from build123d import *

# Parameters (mm, degrees)
SKETCH_1_R          = 1.75
EXTRUDE_1_DEPTH     = 1
SKETCH_2_W          = 5
SKETCH_2_H          = 3.5
SKETCH_2_W_2        = 2
SKETCH_2_H_2        = 6.5
CUT_EXTRUDE_1_DEPTH = 2
SKETCH_3_W          = 14.891608376
SKETCH_3_H          = 2
EXTRUDE_2_DEPTH     = 5
FILLET_1_R          = 2


with BuildPart() as part:
    # 草图1 → 凸台-拉伸1 (new body)
    with BuildSketch(Plane.XY):
        with BuildLine():
            Line((-7.445804188, 14.5), (7.445804188, 14.5))
            ThreePointArc((7.445804188, 14.5), (0, -16.3), (-7.445804188, 14.5))
        make_face()
        Circle(SKETCH_1_R, mode=Mode.SUBTRACT)
    extrude(amount=EXTRUDE_1_DEPTH)

    # 草图2 → 切除-拉伸1 (cut, through all)
    with BuildSketch(Plane.XY.offset(1)):
        with Locations((-16.3, 0)):
            Rectangle(SKETCH_2_W, SKETCH_2_H)
        with Locations((16.2, 0)):
            Rectangle(SKETCH_2_W_2, SKETCH_2_H_2)
    extrude(amount=-CUT_EXTRUDE_1_DEPTH, mode=Mode.SUBTRACT)

    # 草图3 → 凸台-拉伸2 (add)
    with BuildSketch(Plane.XY.offset(1)):
        with Locations((0, 13.5)):
            Rectangle(SKETCH_3_W, SKETCH_3_H)
    extrude(amount=EXTRUDE_2_DEPTH)

    # 圆角1
    fillet_1_edges = [part.edges().sort_by_distance(p)[0] for p in [
        (0, 12.5, 1),
    ]]
    fillet(fillet_1_edges, radius=FILLET_1_R)


solid = part.part
Design review of the part built by this model. Coordinates are the model's own, in mm. A direction names the side the tool comes from. Coordinates: 2 decimals unless noted, no trailing zeros. Loops run counter-clockwise (first coordinate to the right, second up) from the corner with the lowest first, then second, coordinate; pieces in that order, holes last. Notation, with made-up numbers: (89.5, -24) - (97.5, -24) arc R19 cw to (97.5, -14) - close; hole circle Ø1 at (76.5, -23.75). An arc over 180 degrees is marked (long way). Use CSV: the item, a comma, the result in double quotes. Start each with the question number.
1. Add section A-A on x = 0. Give the boundary of the cut face in (y, z).
2. Mouldability with a two-part tool opening along Y and no side actions: class faces 1 (the flat face through (0, -4, 1)), 2 (the flat face through (0, 14.5, 3)), 3 (the flat face through (15.2, 0, 0.5)) as released by +Y, released by -Y, zero draft, split by the parting line, or undercut.
3. Add section C-C on z = 5.3. Give the boundary of the cut face in (x, y).
4. For faces 4 (the flat face through (-7.446, 13, 3)), 5 (the flat face through (7.446, 13, 3)), 6 (the flat face through (0, 12.5, 4)), list the 3-axis set-ups (+Z, -Z, +X, -X, +Y, -Y) from which the entire face can be reached by the end or side of a thin tool; tool diameter is ignored.
5. Add section D-D on x = 6. Give the boundary of the cut face in (y, z), plus the area to 3 significant figures.
6. Add section B-B on y = 0. Give the boundary of the cut face in (x, z), plus the area to 3 significant figures.
7. To check wall thickness, follow probe 1 along Y at (x, z) = (0, 0.45); probe 2 along Z at (x, y) = (8.5, -1); probe 3 along X at (y, z) = (13, 4.2). State the ranges of each line that lie inside material, in increasing order.
8. Clearance check with flat-ended pins moving along their axes: pin 1 (2 mm diameter, centred on x = -8, y = 7.5, fed in from +Z); pin 2 (2 mm diameter, centred on x = 0, y = 0, fed in from -Z); pin 3 (0.9 mm diameter, centred on x = 2.5, z = 4.5, fed in from -Y); pin 4 (2 mm diameter, centred on y = -0.5, z = 1.5, fed in from -X). State where each tip first meets the part, or that it passes through.
Resolved:
1,outline,"(-16.3, 0) - (-1.75, 0) - (-1.75, 1) - (-16.3, 1) - close; (1.75, 0) - (14.5, 0) - (14.5, 6) - (12.5, 6) - (12.5, 3) arc R2 cw to (10.5, 1) - (1.75, 1) - close"
2,face 1,"zero draft"
2,face 2,"released by +Y"
2,face 3,"undercut"
3,outline,"(-7.45, 12.5) - (7.45, 12.5) - (7.45, 14.5) - (-7.45, 14.5) - close"
4,face 4,"+Z, -X, +Y, -Y"
4,face 5,"+Z, +X, +Y, -Y"
4,face 6,"+Z, +X, -X, -Y"
5,outline,"(-15.16, 0) - (14.5, 0) - (14.5, 6) - (12.5, 6) - (12.5, 3) arc R2 cw to (10.5, 1) - (-15.16, 1) - close"
5,area,"40.5 mm2"
6,outline,"(-13.8, 0) - (-1.75, 0) - (-1.75, 1) - (-13.8, 1) - close; (1.75, 0) - (15.2, 0) - (15.2, 1) - (1.75, 1) - close"
6,area,"25.5 mm2"
7,probe 1,"-16.3 to -1.75, 1.75 to 14.5"
7,probe 2,"0 to 1"
7,probe 3,"-7.45 to 7.45"
8,pin 1,"z = 1"
8,pin 2,"through"
8,pin 3,"y = 12.5"
8,pin 4,"x = -13.8"
